```python
from build123d import *

# Parameters (mm, degrees)
F0_W     = 200
F0_H     = 100
F1_DEPTH = 575
F2_R     = 7.5
F3_DEPTH = 20


with BuildPart() as f1:
    # F0 (on Front) → F1 (new body, symmetric)
    with BuildSketch(Plane.XZ):
        with Locations((0, -50)):
            Rectangle(F0_W, F0_H)
        with BuildLine():
            ThreePointArc((-92, -18), (-89.0710678119, -10.9289321881), (-82, -8))
            Line((-82, -8), (82, -8))
            ThreePointArc((82, -8), (89.0710678119, -10.9289321881), (92, -18))
            Line((92, -18), (92, -82))
            ThreePointArc((92, -82), (89.0710678119, -89.0710678119), (82, -92))
            Line((82, -92), (-82, -92))
            ThreePointArc((-82, -92), (-89.0710678119, -89.0710678119), (-92, -82))
            Line((-92, -82), (-92, -18))
        make_face(mode=Mode.SUBTRACT)
    extrude(amount=F1_DEPTH, both=True)

    # F2 (on face) → F3 (join)
    with BuildSketch(Plane.XY):
        with BuildLine():
            Line((-145, -575), (-100, -575))
            Line((-100, -575), (-100, -525))
            Line((-100, -525), (-145, -525))
            ThreePointArc((-145, -525), (-148.5355339059, -526.4644660941), (-150, -530))
            Line((-150, -530), (-150, -570))
            ThreePointArc((-150, -570), (-148.5355339059, -573.5355339059), (-145, -575))
        make_face()
        with Locations((-125, -550)):
            Circle(F2_R, mode=Mode.SUBTRACT)
    extrude(amount=-F3_DEPTH)

    # F4: F1 across plane


with BuildPart() as f1_1:
    add(f1.part)
    add(f1.part.mirror(Plane.XZ))

    # F5: F1 across plane


with BuildPart() as f1_2:
    add(f1_1.part)
    add(f1_1.part.mirror(Plane.YZ))


solid = f1_2.part
```
For this review, take the finished solid that the model builds, in its own axes (mm). A direction names the side the tool comes from. Give positions to 0.01 mm unless a question says otherwise; leave off trailing zeros. Write each loop counter-clockwise with the first axis right and the second up, starting at its lowest first coordinate (ties: lowest second). Pieces come first, ordered by that corner, then holes.
Item 1: Take a section at C-C (y = -428.5). Give the boundary of the cut face in (x, z).
Item 2: Wall thickness on probe 1 along Y at (x, z) = (-125, -8); probe 2 along X at (y, z) = (550, -4.75); probe 3 along X at (y, z) = (-427, -83): over which ranges is each line inside the solid? List them lowest first.
Item 3: Take a section at A-A (x = 60.5). Give the boundary of the cut face in (y, z), and give its area (3 significant figures).
Item 4: Machinability: for faces 4 (the face through (1, -8, -92)), 5 (the face through (-131, -544, -20)), 6 (the face through (131, -544, -20)), 7 (the face through (122, -525, -10)), 8 (the face through (-122, 525, -10)), which of the approach directions +Z, -Z, +X, -X, +Y, -Y give a long, thin tool a straight path to every point of the face, cutting with its end or side? Answer none if there is none.
Item 5: The part is to be moulded in two halves that separate along Z. For faces 1 (the face through (131, 544, -20)), 2 (the face through (122, 525, -10)), 3 (the face through (92, -8, -50)), say which applies: +Z half, -Z half, draft (parallel to the pull), parting line (faces both ways), or undercut.
Item 6: Insertion check: P1, Ø10, axis at y = -251, z = -89.5, coming from the +X side; P2, Ø13.5, axis at x = -125, y = -550, coming from the +Z side; P3, Ø12, axis at x = 22.5, z = -11.5, coming from the -Y side; P4, Ø2, axis at y = 223.5, z = -45.5, coming from the -X side. Each pin has a flat end and moves straight along its axis. Give the tip position at first contact, or say it passes through.
Item 7: Take a section at B-B (z = -31). Give the boundary of the cut face in (x, y), and give its area (3 significant figures).
Established:
1. outline: (-100, -100) - (100, -100) - (100, 0) - (-100, 0) - close; hole (-92, -82) arc R10 ccw to (-82, -92) - (82, -92) arc R10 ccw to (92, -82) - (92, -18) arc R10 ccw to (82, -8) - (-82, -8) arc R10 ccw to (-92, -18) - close
2. probe 1: y = -575 to -557.5, -542.5 to -525, 525 to 542.5, 557.5 to 575
2. probe 2: x = -150 to -132.5, -117.5 to 117.5, 132.5 to 150
2. probe 3: x = -100 to -91.95, 91.95 to 100
3. outline: (-575, -100) - (575, -100) - (575, -92) - (-575, -92) - close; (-575, -8) - (575, -8) - (575, 0) - (-575, 0) - close
3. area: 18,400 mm2
4. face 4: +Y, -Y
4. face 5: -Z, -X, +Y, -Y
4. face 6: -Z, +X, +Y, -Y
4. face 7: +Z, -Z, +X
4. face 8: +Z, -Z, -X
5. face 1: -Z half
5. face 2: draft
5. face 3: undercut
6. P1: stops at x = 100
6. P2: passes through
6. P3: stops at y = -575
6. P4: stops at x = -100
7. outline: (-100, -575) - (-92, -575) - (-92, 575) - (-100, 575) - close; (92, -575) - (100, -575) - (100, 575) - (92, 575) - close
7. area: 18,400 mm2
